from build123d import *

# Parameters (mm, degrees)
CROQUIS1_W              = 25
CROQUIS1_H              = 118
SALIENTE_EXTRUIR1_DEPTH = 25
VACIADO1_T              = -1
CORTAR_EXTRUIR2_DEPTH   = 25
CROQUIS3_W              = 19
CROQUIS3_H              = 20
CORTAR_EXTRUIR3_DEPTH   = 1
CHAFL_N1_SIZE           = 4
CHAFL_N1_SIZE_2         = 6.92820323
CHAFL_N2_SIZE           = 6.92820323
CHAFL_N2_SIZE_2         = 4


with BuildPart() as part:
    # Croquis1 → Saliente-Extruir1 (new body)
    with BuildSketch(Plane.XY):
        with Locations((-22.555898832, -39.876814203)):
            Rectangle(CROQUIS1_W, CROQUIS1_H)
    extrude(amount=SALIENTE_EXTRUIR1_DEPTH)

    # Vaciado1
    vaciado1_openings = [part.faces().sort_by_distance(p)[0] for p in [
        (-22.555898832, -98.876814203, 12.5),
        (-22.555898832, 19.123185797, 12.5),
    ]]
    offset(amount=VACIADO1_T, openings=vaciado1_openings, kind=Kind.INTERSECTION)

    # Croquis2 → Cortar-Extruir2 (cut)
    with BuildSketch(Plane.XY.offset(25)):
        Polygon((-12.555898832, -30.876814203), (-32.555898832, -30.876814203), (-32.555898832, 9.123185797), (-22.555898832, 9.123185797), (-12.555898832, 9.123185797), align=None)
        Polygon((-12.555898832, -88.876814203), (-12.555898832, -48.876814203), (-32.555898832, -48.876814203), (-32.555898832, -88.876814203), (-22.555898832, -88.876814203), align=None)
    extrude(amount=-CORTAR_EXTRUIR2_DEPTH, mode=Mode.SUBTRACT)

    # Croquis3 → Cortar-Extruir3 (cut)
    with BuildSketch(Plane(origin=(-10.055898832, 0, 0), x_dir=(0, 0, -1), z_dir=(1, 0, 0))):
        with Locations((-12.5, -39.876814203)):
            Rectangle(CROQUIS3_W, CROQUIS3_H)
    extrude(amount=-CORTAR_EXTRUIR3_DEPTH, mode=Mode.SUBTRACT)

    # Chaflán1
    # the kernel refuses this chamfer: 6.92820323, 4 mm, written as the material it takes off along each edge
    with BuildSketch(Plane(origin=(-35.055898832, 19.123185797, -17.923855882), x_dir=(0, -1, 0), z_dir=(0, 0, 1))) as chafl_n1_piece_1:
        Polygon((CHAFL_N1_SIZE, 0), (0, CHAFL_N1_SIZE_2), (0, 0), align=None)
    extrude(amount=60.847711765, mode=Mode.SUBTRACT)
    with BuildSketch(Plane(origin=(-10.055898832, 19.123185797, -17.923855882), x_dir=(-1, 0, 0), z_dir=(0, 0, 1))) as chafl_n1_piece_2:
        Polygon((CHAFL_N1_SIZE_2, 0), (0, CHAFL_N1_SIZE), (0, 0), align=None)
    extrude(amount=60.847711765, mode=Mode.SUBTRACT)

    # Chaflán2
    # the kernel refuses this chamfer: 6.92820323, 4 mm, written as the material it takes off along each edge
    with BuildSketch(Plane(origin=(-10.055898832, -98.876814203, -17.923855882), x_dir=(-1, 0, 0), z_dir=(0, 0, 1))) as chafl_n2_piece_1:
        Polygon((CHAFL_N2_SIZE, 0), (0, -CHAFL_N2_SIZE_2), (0, 0), align=None)
    extrude(amount=60.847711765, mode=Mode.SUBTRACT)
    with BuildSketch(Plane(origin=(-35.055898832, -98.876814203, -17.923855882), x_dir=(0, 1, 0), z_dir=(0, 0, 1))) as chafl_n2_piece_2:
        Polygon((CHAFL_N2_SIZE_2, 0), (0, -CHAFL_N2_SIZE), (0, 0), align=None)
    extrude(amount=60.847711765, mode=Mode.SUBTRACT)


solid = part.part
Here's how the part is built. I have some questions about the finished solid (model axes, mm). A direction names the side the tool comes from. Give positions to 0.01 mm unless a question says otherwise; leave off trailing zeros. Write each loop counter-clockwise with the first axis right and the second up, starting at its lowest first coordinate (ties: lowest second). Pieces come first, ordered by that corner, then holes. Notation, with made-up numbers: (-17, 8) -> (14, 8) arc R26 ccw to (14, 35) -> close; hole circle Ø11 at (32, -12.75). An arc over 180 degrees is marked (long way). Use one line per item in the form item = value. Start each with the question number.
1. Imagine slicing it at D-D on x = -29.75. List the corners of the cut face in (y, z) for me.
2. If I drill on L1, parallel to X at y = -32.5, z = 2.5; L2, parallel to Z at x = -21, y = -90.5; L3, parallel to X at y = -42, z = 8.75, over which ranges is the centre line in solid material (lowest first)?
3. Imagine slicing it at B-B on z = 12.5. List the corners of the cut face in (x, y) for me.
4. Will these pins go through, and if not, where does the flat tip stop? pin 1 Ø10 at (x, y) = (-30, -53) entering from -Z; pin 2 Ø0.5 at (x, z) = (-11, 10.5) entering from -Y; pin 3 Ø12 at (x, z) = (-22, 12.5) entering from -Y.
5. Thinking about a two-plate mould opening in X: for faces 3 (the face through (-23, -39, 0)), 4 (the face through (-34.056, -41, 12)), 5 (the face through (-10.056, -41, 23)), which applies, +X half, -X half, draft (parallel to the pull), parting line (faces both ways), or undercut?
6. On a 3-axis mill with a long thin cutter (end or side, diameter ignored), from which of +Z, -Z, +X, -X, +Y, -Y can I reach the whole of each face in a straight line? I mean faces 1 (the face through (-23, -39, 24)), 2 (the face through (-35.056, -41, 12)). Say none if no direction works.
7. Imagine slicing it at C-C on x = -23. List the corners of the cut face in (y, z) for me, plus the area to 3 significant figures.
8. Imagine slicing it at A-A on y = -54. List the corners of the cut face in (x, z) for me.
Entries:
q1.outline = (-97.94, 0) -> (-88.88, 0) -> (-88.88, 1) -> (-97.94, 1) -> close; (-97.94, 24) -> (-88.88, 24) -> (-88.88, 25) -> (-97.94, 25) -> close; (-48.88, 0) -> (-30.88, 0) -> (-30.88, 1) -> (-48.88, 1) -> close; (-48.88, 24) -> (-30.88, 24) -> (-30.88, 25) -> (-48.88, 25) -> close; (9.12, 0) -> (18.19, 0) -> (18.19, 1) -> (9.12, 1) -> close; (9.12, 24) -> (18.19, 24) -> (18.19, 25) -> (9.12, 25) -> close
q2.L1 = -35.06 to -34.06, -11.06 to -10.06
q2.L2 = 0 to 1, 24 to 25
q2.L3 = -35.06 to -34.06
q3.outline = (-35.06, -94.88) -> (-34.06, -95.45) -> (-34.06, 15.7) -> (-35.06, 15.12) -> close; (-11.06, -95.45) -> (-10.06, -94.88) -> (-10.06, -49.88) -> (-11.06, -49.88) -> close; (-11.06, -29.88) -> (-10.06, -29.88) -> (-10.06, 15.12) -> (-11.06, 15.7) -> close
q4.pin_1 = 0
q4.pin_2 = -95.45
q4.pin_3 = through
q5.face_3 = draft
q5.face_4 = undercut
q5.face_5 = +X half
q6.face_1 = +Y, -Y
q6.face_2 = +Z, -Z, -X, +Y, -Y
q7.outline = (-98.88, 0) -> (-88.88, 0) -> (-88.88, 1) -> (-98.88, 1) -> close; (-98.88, 24) -> (-88.88, 24) -> (-88.88, 25) -> (-98.88, 25) -> close; (-48.88, 0) -> (-30.88, 0) -> (-30.88, 1) -> (-48.88, 1) -> close; (-48.88, 24) -> (-30.88, 24) -> (-30.88, 25) -> (-48.88, 25) -> close; (9.12, 0) -> (19.12, 0) -> (19.12, 1) -> (9.12, 1) -> close; (9.12, 24) -> (19.12, 24) -> (19.12, 25) -> (9.12, 25) -> close
q7.area = 76.0 mm²
q8.outline = (-35.06, 0) -> (-32.56, 0) -> (-32.56, 1) -> (-34.06, 1) -> (-34.06, 24) -> (-32.56, 24) -> (-32.56, 25) -> (-35.06, 25) -> close; (-12.56, 0) -> (-10.06, 0) -> (-10.06, 25) -> (-12.56, 25) -> (-12.56, 24) -> (-11.06, 24) -> (-11.06, 1) -> (-12.56, 1) -> close
